Read the model definition and answer for the solid it produces. Units are mm, in the model's axes. Face numbers are marked on the shaded views. A direction names the side the tool comes from. Coordinates: 2 decimals unless noted, no trailing zeros. Loops run counter-clockwise (first coordinate to the right, second up) from the corner with the lowest first, then second, coordinate; pieces in that order, holes last.
Q1. Section D-D (z = 12.5) is taken. Give the vertices of the cut face in (x, y) (3 decimals).
Q2. Straight lines are drawn through the part: line 1 (X direction, y = 25, z = 11); line 2 (Y direction, x = 7, z = 9); line 3 (Y direction, x = 4.5, z = 13). For each, find the intervals that lie inside material, in ascending order.
Q3. Section A-A (y = 31) is taken. Give the vertices of the cut face in (x, z), then the cut area to 3 significant figures.
Q4. Which of the six approach directions +Z, -Z, +X, -X, +Y, -Y give full straight-line access (tool end or side, diameter ignored) to the marked faces 1, 2 and 3?
Q5. Section C-C (x = 7.5) is taken. Give the vertices of the cut face in (y, z).
Q6. Section B-B (z = -22.5) is taken. Give the vertices of the cut face in (x, y).
Q7. Flat-ended cylindrical pins translate along their axes: P1, Ø12, axis at x = 29, z = -5.5, coming from the +Y side; P2, Ø5, axis at x = 29, y = 49, coming from the -Z side; P3, Ø1, axis at x = 55, z = 8.5, coming from the -Y side; P4, Ø10.5, axis at x = 7.5, y = 7.5, coming from the -Z side. Find the tip coordinate at first contact, or state that the pin passes through.
Q8. The mould has two halves that part along Y. Classify the marked faces 4, 5 and 6: pulls with the +Y half, pulls with the -Y half, needs draft (parallel to the pull), parting line crosses it, or undercut.
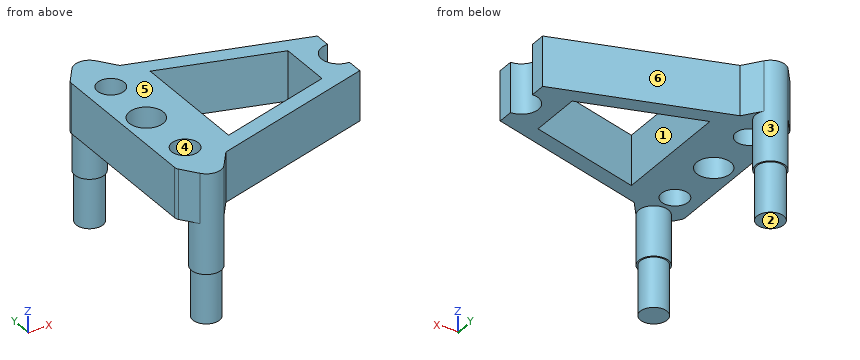
Autodesk Inventor part; units mm, degrees
ref_plane "YZ Plane" through (0, 0, 0) normal (1, 0, 0) x (0, 1, 0)
ref_plane "XZ Plane" through (0, 0, 0) normal (0, 1, 0) x (-1, 0, 0)
ref_plane "XY Plane" through (0, 0, 0) normal (0, 0, 1) x (1, 0, 0)
sketch "Sketch1" plane through (0, 0, 0) normal (0, 0, 1) x (1, 0, 0)
  arc A0 (65, 30.15) -> (65, 19.85) centre (65, 25) ccw
  line L0 (65, 30.15) -> (65, 35)
  line L1 (65, 19.85) -> (65, 15)
  line L2 (65, 25) -> (15, 25)
  line L3 (15, 25) -> (15, 50)
  line L4 (15, 25) -> (15, 0)
  line L5 (15, 0) -> (65, 15)
  line L6 (15, 50) -> (65, 35)
  line L7 (15, 50) -> (0, 50)
  line L8 (0, 50) -> (0, 0)
  line L9 (0, 0) -> (15, 0)
  line L10 (15, 25) -> (20, 25)
  line L11 (20, 25) -> (20, 48.5)
  line L12 (20, 25) -> (20, 1.5)
  line L13 (59.85, 25) -> (54.85, 25)
  line L14 (54.85, 25) -> (54.85, 38.045)
  line L15 (54.85, 25) -> (54.85, 11.955)
  line L16 (20, 1.5) -> (20, 6.5)
  line L17 (20, 6.5) -> (54.85, 16.955)
  line L18 (20, 48.5) -> (20, 43.5)
  line L19 (20, 43.5) -> (54.85, 33)
  line L20 (7.5, 50) -> (7.5, 0)
  line L21 (0, 25) -> (15, 25)
  line L22 (0, 50) -> (15, 35)
  line L23 (0, 50) -> (21.2132, 50) construction
  line L24 (0, 0) -> (15, 15)
  line L25 (0, 0) -> (21.2132, 0) construction
  circle A1 centre (7.5, 7.5) radius 4.05
  circle A2 centre (7.5, 42.5) radius 4.05
  line L26 (65, 19.85) -> (65, 25)
  line L27 (65, 30.15) -> (65, 25)
  line L28 (7.5, 25) -> (7, 25)
  circle A3 centre (7, 25) radius 5.15
  line L29 (0, 50) -> (15, 50)
  line L30 (15, 50) -> (15, 60)
  line L31 (15, 60) -> (0, 60)
  line L32 (0, 60) -> (0, 50)
  line L33 (15, 0) -> (0, 0)
  line L34 (0, 0) -> (0, -10)
  line L35 (0, -10) -> (15, -10)
  line L36 (15, -10) -> (15, 0)
  line L37 (7.5, -10) -> (7.5, -2.5)
  line L38 (7.5, 60) -> (7.5, 52.5)
  circle A4 centre (7.5, 52.5) radius 4.05
  circle A5 centre (7.5, 52.5) radius 4.5
  circle A6 centre (7.5, -2.5) radius 4.05
  circle A7 centre (7.5, -2.5) radius 4.5
  line L39 (0, 50) -> (3.9, 55.2)
  line L40 (15, 50) -> (11.1, 55.2)
  line L41 (0, 0) -> (3.9, -5.2)
  line L42 (15, 0) -> (11.1, -5.2)
  point P0 (0, 0)
  point P1 (3.7583, 0)
  point P2 (11.2417, 0)
  point P3 (11.2417, 50)
  point P4 (3.7583, 50)
  point P5 (0, 0)
  dimension "d0" = 10.3
  dimension "d1" = 50
  dimension "d2" = 25
  dimension "d3" = 25
  dimension "d4" = 15
  dimension "d5" = 50
  dimension "d6" = 90
  dimension "d7" = 5
  dimension "d8" = 5
  dimension "d9" = 5
  dimension "d10" = 5
  dimension "d11" = 45
  dimension "d12" = 45
  dimension "d13" = 8.1
  dimension "d14" = 8.1
  dimension "d15" = 50
  dimension "d16" = 10
  dimension "d17" = 20
  dimension "d18" = 10
  dimension "d19" = 5.045
  dimension "d46" = 0.5
  dimension "d47" = 10.3
  dimension "d48" = 15
  dimension "d49" = 10
  dimension "d50" = 15
  dimension "d51" = 10
  dimension "d52" = 7.5
  dimension "d53" = 7.5
  dimension "d54" = 8.1
  dimension "d55" = 9
  dimension "d56" = 8.1
  dimension "d57" = 9
extrude "Extrusion1" add sketch "Sketch1" along normal blind 15 contours A0 L2 L14 L6 L0 | A0 L1 L5 L15 L2 | L14 L19 L11 L6 | L12 L5 L4 L2 | L2 L3 L6 L11 | L15 L5 L12 L17 | L21 A3 L20 A2 L22 L3 | L4 L24 A1 L20 A3 L21 | L3 L22 A2 L20 A5 L7 | L7 A5 L40 | L4 L9 A7 L20 A1 L24 | A5 L20 A4 L7 | L7 A4 L38 A5 | L42 A7 L9 | A3 L21 L8 L22 A2 L20 | L20 A1 L24 L8 L21 A3 | A4 L20 L7 | L7 A4 | A5 L7 A4 L20 | L20 A2 L22 L7 A5 | L38 A4 L7 A5 | A7 L37 A6 L9 | L9 A6 L20 A7 | L20 A4 L7 | L7 L39 A5 | A6 L9 | L9 L20 A6 | A7 L9 L24 A1 L20 | L20 A6 L9 A7 | A7 L9 A6 L37 | L9 A6 L20 | A7 L41 L9
extrude "Extrusion2" add sketch "Sketch1" against normal blind 15 contours A5 L20 A4 L7 | L7 A4 L38 A5 | A4 L20 L7 | L7 A4 | A5 L7 A4 L20 | L38 A4 L7 A5 | A7 L37 A6 L9 | L9 A6 L20 A7 | L20 A4 L7 | A6 L9 | L9 L20 A6 | L20 A6 L9 A7 | A7 L9 A6 L37 | L9 A6 L20
extrude "Extrusion3" add sketch "Sketch1" against normal blind 30 contours A4 L20 L7 | L7 A4 | L20 A4 L7 | A6 L9 | L9 L20 A6 | L9 A6 L20
fillet "Fillet1" radius 2 2 edges at (0, 0, 7.5) (0, 50, 7.5)
properties part number "Rod_support_2"
Numbers:
1. outline: (0, 0.667) arc R2 ccw to (0.4, -0.533) - (3.9, -5.2) arc R4.5 ccw to (11.1, -5.2) - (15, 0) - (65, 15) - (65, 19.85) arc R5.15 cw to (65, 30.15) - (65, 35) - (15, 50) - (11.1, 55.2) arc R4.5 ccw to (3.9, 55.2) - (0.4, 50.533) arc R2 ccw to (0, 49.333) - close; hole circle Ø10.3 at (7, 25); hole circle Ø8.1 at (7.5, 7.5); hole circle Ø8.1 at (7.5, 42.5); hole (20, 6.5) - (54.85, 16.955) - (54.85, 33) - (20, 43.5) - close
2. line 1: x = 0 to 1.85, 12.15 to 20, 54.85 to 59.85
2. line 2: y = -6.97 to 3.48, 11.52 to 19.85, 30.15 to 38.48, 46.52 to 56.97
2. line 3: y = -5.85 to 4.78, 10.22 to 20.5, 29.5 to 39.78, 45.22 to 55.85
3. outline: (0, 0) - (20, 0) - (20, 15) - (0, 15) - close; (54.85, 0) - (65, 0) - (65, 15) - (54.85, 15) - close
3. area: 452 mm2
4. face 1: +Z, -Z
4. face 2: -Z, +X, -X, +Y, -Y
4. face 3: -Z
5. outline: (-7, -15) - (-6.55, -15) - (-6.55, -30) - (1.55, -30) - (1.55, -15) - (2, -15) - (2, 0) - (3.45, 0) - (3.45, 15) - (-7, 15) - close; (11.55, 0) - (19.87, 0) - (19.87, 15) - (11.55, 15) - close; (30.13, 0) - (38.45, 0) - (38.45, 15) - (30.13, 15) - close; (46.55, 0) - (48, 0) - (48, -15) - (48.45, -15) - (48.45, -30) - (56.55, -30) - (56.55, -15) - (57, -15) - (57, 15) - (46.55, 15) - close
6. outline: circle Ø8.1 at (7.5, -2.5); circle Ø8.1 at (7.5, 52.5)
7. P1: stops at y = 46.52
7. P2: passes through
7. P3: stops at y = 11.85
7. P4: stops at z = 0
8. face 4: undercut
8. face 5: needs draft
8. face 6: pulls with the +Y half
